```python
from build123d import *

# Parameters (mm, degrees)
F1_DEPTH = 38.1
F3_DEPTH = 12.7
F4_R     = 6.35
F4_R_2   = 4.745300615
F5_DEPTH = 38.101


# Not quite as in the source:
# - a feature names something its author has since deleted; it is built from what else it names


with BuildPart() as f1:
    # F0 (on Front) → F1 (new body)
    with BuildSketch(Plane.XZ):
        Polygon((0, 38.1), (0, 0), (38.1, 0), (38.1, 12.7), (69.85, 12.7), (69.85, 25.4), (38.1, 25.4), (38.1, 38.1), align=None)
    extrude(amount=F1_DEPTH)

    # F2 (on face) → F3 (join)
    with BuildSketch(Plane.XY.offset(25.4)):
        with BuildLine():
            Line((69.85, 0), (69.85, -38.1))
            ThreePointArc((69.85, -38.1), (88.9, -19.05), (69.85, 0))
        make_face()
    extrude(amount=-F3_DEPTH)

    # F4 (on face) → F5 (cut, through all)
    with BuildSketch(Plane.XY.offset(38.1)):
        with Locations((19.05, -19.6927841753)):
            Circle(F4_R)
        with Locations((50.8, -12.7)):
            Circle(F4_R_2)
        with Locations((50.8, -25.4)):
            Circle(F4_R_2)
        with Locations((69.85, -25.4)):
            Circle(F4_R_2)
        with Locations((69.85, -12.7)):
            Circle(F4_R_2)
    extrude(amount=-F5_DEPTH, mode=Mode.SUBTRACT)


solid = f1.part
```
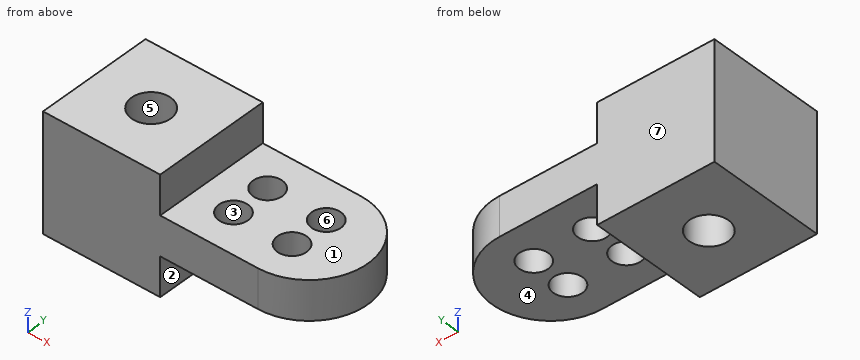
Could you check a few things on this model? Use its own coordinates, in mm. Face numbers are marked on the shaded views. A direction names the side the tool comes from. Give positions to 0.01 mm unless a question says otherwise; leave off trailing zeros. Order: outer loops, then holes, each group sorted by start corner. A loop starts at its lowest first (then second) coordinate and runs counter-clockwise, first axis right, second up.
Q1. Suppose I cut it at C-C, the plane x = 50.8. Write out the boundary of the cut face in (y, z), and give its area (3 significant figures).
Q2. Suppose I cut it at A-A, the plane x = 19.05. Write out the boundary of the cut face in (y, z), and give its area (3 significant figures).
Q3. We'd pull the mould along Y, two halves only. Please class the marked faces 4, 5, 6 and 7: +Y half, -Y half, draft (parallel to the pull), parting line (faces both ways), or undercut.
Q4. Suppose I cut it at B-B, the plane y = -15. Write out the boundary of the cut face in (x, z).
Q5. I'm going to push flat-ended pins straight in: P1, Ø12.5, axis at x = 69.85, y = -12.7, coming from the -Z side; P2, Ø4, axis at y = -17, z = 34.5, coming from the +X side; P3, Ø8.5, axis at x = 50.8, y = -12.7, coming from the +Z side; P4, Ø11.5, axis at x = 56.5, y = -25, coming from the +Z side. Where does each tip first touch, or does it pass through?
Q6. For the marked faces 1, 2 and 3, which set-ups out of +Z, -Z, +X, -X, +Y, -Y let a thin tool reach every point of the face, with its end or its side?
Q7. If I drill on line 1 along Y through (x, z) = (69.85, 21); line 2 along X through (y, z) = (-20, 33.5); line 3 along Y through (x, z) = (52, 24), over which ranges is the centre line in solid material (lowest first)?
Q8. Suppose I cut it at D-D, the plane y = -27.5. Write out the boundary of the cut face in (x, z).
Solution:
1. outline: (-38.1, 12.7) - (-30.15, 12.7) - (-30.15, 25.4) - (-38.1, 25.4) - close; (-20.65, 12.7) - (-17.45, 12.7) - (-17.45, 25.4) - (-20.65, 25.4) - close; (-7.95, 12.7) - (0, 12.7) - (0, 25.4) - (-7.95, 25.4) - close
1. area: 243 mm2
2. outline: (-38.1, 0) - (-26.04, 0) - (-26.04, 38.1) - (-38.1, 38.1) - close; (-13.34, 0) - (0, 0) - (0, 38.1) - (-13.34, 38.1) - close
2. area: 968 mm2
3. face 4: draft
3. face 5: undercut
3. face 6: undercut
3. face 7: +Y half
4. outline: (0, 0) - (14.77, 0) - (14.77, 38.1) - (0, 38.1) - close; (23.33, 0) - (38.1, 0) - (38.1, 12.7) - (46.65, 12.7) - (46.65, 25.4) - (38.1, 25.4) - (38.1, 38.1) - (23.33, 38.1) - close; (54.95, 12.7) - (65.7, 12.7) - (65.7, 25.4) - (54.95, 25.4) - close; (74, 12.7) - (88.46, 12.7) - (88.46, 25.4) - (74, 25.4) - close
5. P1: stops at z = 12.7
5. P2: stops at x = 38.1
5. P3: passes through
5. P4: stops at z = 25.4
6. face 1: +Z, +X, +Y, -Y
6. face 2: -Z, +X, +Y, -Y
6. face 3: +Z, -Z
7. line 1: y = -38.1 to -30.15, -20.65 to -17.45, -7.95 to 0
7. line 2: x = 0 to 12.71, 25.39 to 38.1
7. line 3: y = -38.1 to -29.99, -20.81 to -17.29, -8.11 to 0
8. outline: (0, 0) - (38.1, 0) - (38.1, 12.7) - (46.54, 12.7) - (46.54, 25.4) - (38.1, 25.4) - (38.1, 38.1) - (0, 38.1) - close; (55.06, 12.7) - (65.59, 12.7) - (65.59, 25.4) - (55.06, 25.4) - close; (74.11, 12.7) - (86.92, 12.7) - (86.92, 25.4) - (74.11, 25.4) - close
